```python
from build123d import *

# Parameters (mm, degrees)
SKETCH1_R           = 1.55
BOSS_EXTRUDE1_DEPTH = 6


with BuildPart() as part:
    # Sketch1 → Boss-Extrude1 (new body)
    with BuildSketch(Plane(origin=(0, 0, 0), x_dir=(1, 0, 0), z_dir=(0, 1, 0))):
        with BuildLine():
            Line((-22.5, -5), (-22.5, -22.5))
            Line((-22.5, -22.5), (22.5, -22.5))
            Line((22.5, -22.5), (22.5, -5))
            Line((22.5, -5), (17.5, -5))
            ThreePointArc((17.5, -5), (12.5, 0), (17.5, 5))
            Line((17.5, 5), (22.5, 5))
            Line((22.5, 5), (22.5, 22.5))
            Line((22.5, 22.5), (-22.5, 22.5))
            Line((-22.5, 22.5), (-22.5, 5))
            Line((-22.5, 5), (-17.5, 5))
            ThreePointArc((-17.5, 5), (-12.5, 0), (-17.5, -5))
            Line((-17.5, -5), (-22.5, -5))
        make_face()
        with Locations(Location((-18.65, -18.65, 0), (0, 0, 270))):
            Circle(SKETCH1_R, mode=Mode.SUBTRACT)
        with Locations(Location((18.65, -18.65, 0), (0, 0, 270))):
            Circle(SKETCH1_R, mode=Mode.SUBTRACT)
        with Locations(Location((-18.65, 18.65, 0), (0, 0, 270))):
            Circle(SKETCH1_R, mode=Mode.SUBTRACT)
        with Locations(Location((18.65, 18.65, 0), (0, 0, 270))):
            Circle(SKETCH1_R, mode=Mode.SUBTRACT)
    extrude(amount=BOSS_EXTRUDE1_DEPTH)


solid = part.part
```
Check sheet for the modelled part. Datum: model origin and axes. Units: mm. A direction names the side the tool comes from. Give positions to 0.01 mm unless a question says otherwise; leave off trailing zeros. Order: outer loops, then holes, each group sorted by start corner. A loop starts at its lowest first (then second) coordinate and runs counter-clockwise, first axis right, second up. Notation, with made-up numbers: M 69,10 L 105,10 A8 cw 105,23 Z; hole C 8.25,61 d4. An arc over 180 degrees is marked long. Answer in a Markdown table with one row per item.
1) Cross-section at A-A, the plane x = 18.65. Enter the section's corners in (y, z).
Filled sheet:
| item | result |
|---|---|
| outline | M 0,-22.5 L 6,-22.5 L 6,-20.2 L 0,-20.2 Z; M 0,-17.1 L 6,-17.1 L 6,-5 L 0,-5 Z; M 0,5 L 6,5 L 6,17.1 L 0,17.1 Z; M 0,20.2 L 6,20.2 L 6,22.5 L 0,22.5 Z |
2) Gauge pin test, flat end, axial feed: P1, Ø1.5, axis at y = 3.5, z = 0.5, coming from the -X side. Record the tip position at first contact, or that the pin passes through.
Filled sheet:
| item | result |
|---|---|
| P1 | stops at x = -12.66 |
3) Access from +Z, -Z, +X, -X, +Y, -Y to the whole of each face (thin tool, end or side, straight path). Record for faces 4 (the cylindrical face through (18.1, 3, 20.1)), 5 (the flat face through (-20, 3, 5)), 6 (the flat face through (20, 3, 5)).
Filled sheet:
| item | result |
|---|---|
| face 4 | +Y, -Y |
| face 5 | -X, +Y, -Y |
| face 6 | +X, +Y, -Y |
4) Cross-section at B-B, the plane y = 0.55. Enter the section's corners in (x, z).
Filled sheet:
| item | result |
|---|---|
| outline | M -22.5,-22.5 L 22.5,-22.5 L 22.5,-5 L 17.5,-5 A5 cw 17.5,5 L 22.5,5 L 22.5,22.5 L -22.5,22.5 L -22.5,5 L -17.5,5 A5 cw -17.5,-5 L -22.5,-5 Z; hole C -18.65,-18.65 d3.1; hole C -18.65,18.65 d3.1; hole C 18.65,-18.65 d3.1; hole C 18.65,18.65 d3.1 |
5) Thickness scan on L1, parallel to X at y = 1.85, z = -18.65; L2, parallel to X at y = 1.45, z = -19.5; L3, parallel to X at y = 4, z = 1.5. Record the ranges inside material, lowest first. Write a range as [from, to].
Filled sheet:
| item | result |
|---|---|
| L1 | x = [-22.5, -20.2], [-17.1, 17.1], [20.2, 22.5] |
| L2 | x = [-22.5, -19.95], [-17.35, 17.35], [19.95, 22.5] |
| L3 | x = [-12.73, 12.73] |
6) Release check for a two-part mould opening along X. For faces 1 (the flat face through (22.5, 3, 14)), 2 (the cylindrical face through (18.1, 3, -17.2)), 3 (the flat face through (0, 6, 0)) record: +X half, -X half, draft (parallel to the pull), parting line (faces both ways), or undercut.
Filled sheet:
| item | result |
|---|---|
| face 1 | +X half |
| face 2 | undercut |
| face 3 | draft |
7) Cross-section at D-D, the plane x = 13.5. Enter the section's corners in (y, z), plus the area to 3 significant figures.
Filled sheet:
| item | result |
|---|---|
| outline | M 0,-22.5 L 6,-22.5 L 6,-3 L 0,-3 Z; M 0,3 L 6,3 L 6,22.5 L 0,22.5 Z |
| area | 234 mm2 |
8) Cross-section at C-C, the plane z = -18.65. Enter the section's corners in (x, y), plus the area to 3 significant figures.
Filled sheet:
| item | result |
|---|---|
| outline | M -22.5,0 L -20.2,0 L -20.2,6 L -22.5,6 Z; M -17.1,0 L 17.1,0 L 17.1,6 L -17.1,6 Z; M 20.2,0 L 22.5,0 L 22.5,6 L 20.2,6 Z |
| area | 233 mm2 |
